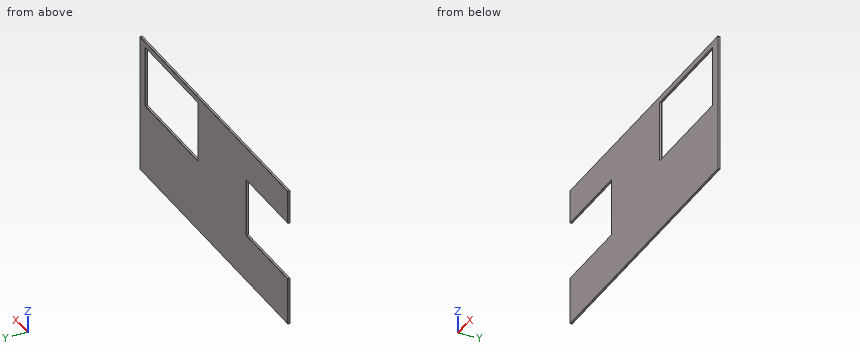
```python
from build123d import *

# Parameters (mm, degrees)
SKETCH1_W           = 869.95
SKETCH1_H           = 534.924
BOSS_EXTRUDE1_DEPTH = 19.05
CHAMFER1_SIZE       = 2.54


with BuildPart() as part:
    # Sketch1 → Boss-Extrude1 (new body)
    with BuildSketch(Plane(origin=(0, 0, 0), x_dir=(1, 0, 0), z_dir=(0, 1, 0))):
        Polygon((2438.4, 0), (2438.4, 1219.2), (0, 1219.2), (0, 803.275), (685.8, 803.275), (685.8, 295.275), (0, 295.275), (0, 0), align=None)
        with Locations((1914.4615, 318.262)):
            Rectangle(SKETCH1_W, SKETCH1_H, mode=Mode.SUBTRACT)
    extrude(amount=-BOSS_EXTRUDE1_DEPTH)

    # Chamfer1
    chamfer1_edges = [part.edges().sort_by_distance(p)[0] for p in [
        (0, 0, -1011.2375),
        (1219.2, 0, -1219.2),
        (2438.4, 0, -609.6),
        (1219.2, 0, 0),
        (1914.4615, 0, -585.724),
        (1479.4865, 0, -318.262),
        (1914.4615, 0, -50.8),
        (2349.4365, 0, -318.262),
        (0, 0, -147.6375),
        (342.9, 0, -295.275),
        (685.8, 0, -549.275),
        (342.9, 0, -803.275),
    ]]
    chamfer(chamfer1_edges, length=CHAMFER1_SIZE)


solid = part.part
```
Here's how the part is built. I have some questions about the finished solid (model axes, mm). Coordinates: 2 decimals unless noted, no trailing zeros. Loops run counter-clockwise (first coordinate to the right, second up) from the corner with the lowest first, then second, coordinate; pieces in that order, holes last. Notation, with made-up numbers: (79.25, -9) - (122.25, -9) arc R27 cw to (122.25, 21) - close; hole circle Ø6 at (83.5, 44.25). An arc over 180 degrees is marked (long way). Return JSON: item names as keys, results as strings. Group by question number.
Item 1: If we section it at C-C on y = -9.5: Write out the boundary of the cut face in (x, z) (1 decimal), and give its area (3 significant figures).
Item 2: Will this pin go through, and if not, where does the flat tip stop? P1, Ø2, axis at y = -9.5, z = -525, coming from the -X side.
Item 3: If we section it at B-B on z = -250.5: Write out the boundary of the cut face in (x, y).
Item 4: I need wall thicknesses on line 1 (Z direction, x = 2057.5, y = -5); line 2 (X direction, y = -2.25, z = -80.5); line 3 (X direction, y = -2.5, z = -259). Which ranges of each line are inside material? Lowest first, please. Write a range as from..to.
Item 5: If we section it at A-A on x = 522.5: Write out the boundary of the cut face in (y, z) (3 decimals).
Calculated:
{
 "1": {"outline": "(0, -1219.2) - (2438.4, -1219.2) - (2438.4, 0) - (0, 0) - (0, -295.3) - (685.8, -295.3) - (685.8, -803.3) - (0, -803.3) - close; hole (1479.5, -585.7) - (2349.4, -585.7) - (2349.4, -50.8) - (1479.5, -50.8) - close", "area": "2,160,000 mm^2"},
 "2": {"P1": "stops at x = 685.8"},
 "3": {"outline": "(0, -19.05) - (1479.49, -19.05) - (1479.49, -2.54) - (1476.95, 0) - (2.54, 0) - (0, -2.54) - close; (2349.44, -19.05) - (2438.4, -19.05) - (2438.4, -2.54) - (2435.86, 0) - (2351.98, 0) - (2349.44, -2.54) - close"},
 "4": {"line 1": "z = -1219.2..-585.72, -50.8..0", "line 2": "x = 0.29..1479.2, 2349.73..2438.11", "line 3": "x = 0.04..1479.45, 2349.48..2438.36"},
 "5": {"outline": "(-19.05, -1219.2) - (-2.54, -1219.2) - (0, -1216.66) - (0, -805.815) - (-2.54, -803.275) - (-19.05, -803.275) - close; (-19.05, -295.275) - (-2.54, -295.275) - (0, -292.735) - (0, -2.54) - (-2.54, 0) - (-19.05, 0) - close"}
}
